Check sheet for the modelled part. Datum: model origin and axes. Units: mm. A direction names the side the tool comes from. Give positions to 0.01 mm unless a question says otherwise; leave off trailing zeros. Loops run counter-clockwise (first coordinate to the right, second up) from the corner with the lowest first, then second, coordinate; pieces in that order, holes last. Notation, with made-up numbers: (73, 29.25) -> (88, 29.25) arc R20 cw to (88, 47.25) -> close; hole circle Ø6 at (-39.75, 45). An arc over 180 degrees is marked (long way). Answer as CSV lines item,"result". Start each with the question number.
(1) Section check B-B on x = 0. Enter the section's corners in (y, z) (3 decimals).
(2) Release check for a two-part mould opening along Z. For faces 1 (the face through (2, 8, -4)), 2 (the face through (7.808, 3.944, -1.025)), 3 (the face through (-2.44, 3.99, 0.54)) record: pulls with the +Z half, pulls with the -Z half, needs draft (parallel to the pull), parting line crosses it, or undercut.
(3) Gauge pin test, flat ends, axial feed: pin 1 Ø1 at (y, z) = (1.5, -3.5) entering from -X; pin 2 Ø5.5 at (x, z) = (1, 0) entering from -Y; pin 3 Ø1 at (x, y) = (4, 2) entering from -Z. Record the tip position at first contact, or that the pin passes through.
(4) Material ranges on line 1 (X direction, y = 2.3, z = 0) (3 decimals); line 2 (X direction, y = 5.45, z = 0) (3 decimals); line 3 (Z direction, x = -0.25, y = 7), recorded low to high. Write a range as from..to.
(5) Section check D-D on y = 0.75. Enter the section's corners in (x, z) (3 decimals), plus the area to 3 significant figures.
(6) Section check C-C on y = 4.25. Enter the section's corners in (x, z) (3 decimals), plus the area to 3 significant figures.
(7) Access from +Z, -Z, +X, -X, +Y, -Y to the whole of each face (thin tool, end or side, straight path). Record for faces 4 (the face through (2, 5, -1)), 5 (the face through (2, 0, -4)).
(8) Section check A-A on z = 0. Enter the section's corners in (x, y) (3 decimals), plus the area to 3 significant figures.
from build123d import *

# Parameters (mm, degrees)
SKETCH1_R           = 7.875
SKETCH1_R_2         = 1.75
BOSS_EXTRUDE1_DEPTH = 8
SKETCH2_R           = 4
CUT_EXTRUDE1_DEPTH  = 3
CUT_EXTRUDE1_DRAFT  = -45
SKETCH3_R           = 4
CUT_EXTRUDE2_DEPTH  = 5
BOSS_EXTRUDE2_START = 2
SKETCH4_R           = 4
SKETCH4_R_2         = 2.5
BOSS_EXTRUDE2_DEPTH = 2


with BuildPart() as part:
    # Sketch1 → Boss-Extrude1 (new body)
    with BuildSketch(Plane(origin=(0, 0, 0), x_dir=(1, 0, 0), z_dir=(0, 1, 0))):
        with Locations(Location((0, 0, 0), (0, 0, 270))):
            Circle(SKETCH1_R)
        with Locations(Location((0, 0, 0), (0, 0, 270))):
            Circle(SKETCH1_R_2, mode=Mode.SUBTRACT)
    extrude(amount=BOSS_EXTRUDE1_DEPTH)


with BuildPart() as cut_extrude1_tool:
    # Sketch2 → Cut-Extrude1 (with draft: the straight prism first)
    with BuildSketch(Plane(origin=(0, 8, 0), x_dir=(1, 0, 0), z_dir=(0, 1, 0))):
        Circle(SKETCH2_R)
    extrude(amount=-CUT_EXTRUDE1_DEPTH)
    # Cut-Extrude1: the draft: its side faces are tilted about the plane it starts from
    cut_extrude1_sides = [cut_extrude1_tool.faces().sort_by_distance(p)[0] for p in [
        (-4, 6.5, 0),
    ]]
    draft(cut_extrude1_sides, Plane(origin=(0, 8, 0), x_dir=(1, 0, 0), z_dir=(0, 1, 0)), CUT_EXTRUDE1_DRAFT)


with BuildPart() as part_1:
    add(part.part)

    # Cut-Extrude1: cut by cut_extrude1_tool
    add(cut_extrude1_tool.part, mode=Mode.SUBTRACT)

    # Sketch3 → Cut-Extrude2 (cut)
    with BuildSketch(Plane(origin=(0, 0, 0), x_dir=(-1, 0, 0), z_dir=(0, -1, 0))):
        with Locations(Location((0, 0, 0), (0, 0, 90))):
            Circle(SKETCH3_R)
    extrude(amount=-CUT_EXTRUDE2_DEPTH, mode=Mode.SUBTRACT)

    # Sketch4 → Boss-Extrude2 (add)
    with BuildSketch(Plane.XZ.offset(-5).offset(BOSS_EXTRUDE2_START)):
        with Locations(Location((0, 0, 0), (0, 0, 270))):
            Circle(SKETCH4_R)
        with Locations(Location((0, 0, 0), (0, 0, 270))):
            Circle(SKETCH4_R_2, mode=Mode.SUBTRACT)
    extrude(amount=-BOSS_EXTRUDE2_DEPTH)


solid = part_1.part
Working result:
1,outline,"(0, -7.875) -> (8, -7.875) -> (8, -4) -> (5.75, -1.75) -> (5, -1.75) -> (5, -2.5) -> (3, -2.5) -> (3, -4) -> (0, -4) -> close; (0, 4) -> (3, 4) -> (3, 2.5) -> (5, 2.5) -> (5, 1.75) -> (5.75, 1.75) -> (8, 4) -> (8, 7.875) -> (0, 7.875) -> close"
2,face 1,"needs draft"
2,face 2,"parting line crosses it"
2,face 3,"undercut"
3,pin 1,"stops at x = -7.28"
3,pin 2,"stops at y = 3"
3,pin 3,"stops at z = -7.05"
4,line 1,"x = -7.875..-4, 4..7.875"
4,line 2,"x = -7.875..-1.75, 1.75..7.875"
4,line 3,"z = -7.87..-2.99, 2.99..7.87"
5,outline,"circle Ø15.75 at (0, 0); hole circle Ø8 at (0, 0)"
5,area,"145 mm^2"
6,outline,"circle Ø15.75 at (0, 0); hole circle Ø5 at (0, 0)"
6,area,"175 mm^2"
7,face 4,"-Y"
7,face 5,"+Z, -Z, +X, -X, -Y"
8,outline,"(-7.875, 0) -> (-4, 0) -> (-4, 3) -> (-2.5, 3) -> (-2.5, 5) -> (-1.75, 5) -> (-1.75, 5.75) -> (-4, 8) -> (-7.875, 8) -> close; (1.75, 5) -> (2.5, 5) -> (2.5, 3) -> (4, 3) -> (4, 0) -> (7.875, 0) -> (7.875, 8) -> (4, 8) -> (1.75, 5.75) -> close"
8,area,"76.4 mm^2"
